For this review, take the finished solid that the model builds, in its own axes (mm). A direction names the side the tool comes from. Round coordinates to 2 decimals unless told otherwise and drop trailing zeros. Order: outer loops, then holes, each group sorted by start corner. A loop starts at its lowest first (then second) coordinate and runs counter-clockwise, first axis right, second up. Notation, with made-up numbers: M 44.25,-13 L 94.25,-13 A14 cw 94.25,12 Z; hole C -23.75,30 d6. An arc over 180 degrees is marked long. Answer as a JSON object with one key per item and string values.
from build123d import *

# Parameters (mm, degrees)
SKETCH1_W           = 7
SKETCH1_H           = 7
BOSS_EXTRUDE1_DEPTH = 4
CUT_EXTRUDE1_DEPTH  = 2
SKETCH4_R           = 1.45
CUT_EXTRUDE2_DEPTH  = 2
FILLET1_R           = 2


with BuildPart() as part:
    # Sketch1 → Boss-Extrude1 (new body)
    with BuildSketch(Plane(origin=(0, 0, 0), x_dir=(1, 0, 0), z_dir=(0, 1, 0))):
        Rectangle(SKETCH1_W, SKETCH1_H)
    extrude(amount=BOSS_EXTRUDE1_DEPTH)

    # Sketch2 → Cut-Extrude1 (cut)
    with BuildSketch(Plane(origin=(0, 4, 0), x_dir=(1, 0, 0), z_dir=(0, 1, 0))):
        Polygon((2.598076211, -1.5), (2.598076211, 1.5), (0, 3), (-2.598076211, 1.5), (-2.598076211, -1.5), (0, -3), align=None)
    extrude(amount=-CUT_EXTRUDE1_DEPTH, mode=Mode.SUBTRACT)

    # Sketch4 → Cut-Extrude2 (cut)
    with BuildSketch(Plane(origin=(0, 2, 0), x_dir=(1, 0, 0), z_dir=(0, 1, 0))):
        with Locations(Location((0, 0, 0), (0, 0, 270))):
            Circle(SKETCH4_R)
    extrude(amount=-CUT_EXTRUDE2_DEPTH, mode=Mode.SUBTRACT)

    # Fillet1
    fillet1_edges = [part.edges().sort_by_distance(p)[0] for p in [
        (3.5, 2, 3.5),
        (-3.5, 2, 3.5),
        (-3.5, 2, -3.5),
        (3.5, 2, -3.5),
    ]]
    fillet(fillet1_edges, radius=FILLET1_R)


solid = part.part
1) Machinability: for faces 1 (the flat face through (2.598, 3, 0)), 2 (the flat face through (-3.5, 2, 0)), which of the approach directions +Z, -Z, +X, -X, +Y, -Y give a long, thin tool a straight path to every point of the face, cutting with its end or side? Answer none if there is none.
Geometry check:
{"face 1": "+Y", "face 2": "+Z, -Z, -X, +Y, -Y"}
2) Add section A-A on z = 0. State the section outline as (x, y) points, and give its area (3 significant figures).
Geometry check:
{"outline": "M -3.5,0 L -1.45,0 L -1.45,2 L -2.6,2 L -2.6,4 L -3.5,4 Z; M 1.45,0 L 3.5,0 L 3.5,4 L 2.6,4 L 2.6,2 L 1.45,2 Z", "area": "11.8 mm²"}
3) For L1, parallel to X at y = 0.75, z = 0; L2, parallel to X at y = 2.25, z = -0.75; L3, parallel to Y at x = 1.25, z = 2, list the stretches that pass through material, from the lowest coordinate up.
Geometry check:
{"L1": "x = -3.5 to -1.45, 1.45 to 3.5", "L2": "x = -3.5 to -2.6, 2.6 to 3.5", "L3": "y = 0 to 2"}
4) Add section B-B on y = 1.4. State the section outline as (x, z) points.
Geometry check:
{"outline": "M -3.5,-1.5 A2 ccw -1.5,-3.5 L 1.5,-3.5 A2 ccw 3.5,-1.5 L 3.5,1.5 A2 ccw 1.5,3.5 L -1.5,3.5 A2 ccw -3.5,1.5 Z; hole C 0,0 d2.9"}
5) Mouldability with a two-part tool opening along X and no side actions: class faces 3 (the flat face through (1.1, 2, 1.3)), 4 (the cylindrical face through (-2.93, 2.03, -2.9)), 5 (the flat face through (0, 2, -3.5)) as +X half, -X half, draft (parallel to the pull), parting line (faces both ways), or undercut.
Geometry check:
{"face 3": "undercut", "face 4": "-X half", "face 5": "draft"}
6) Add section C-C on x = 0.75. State the section outline as (y, z) points.
Geometry check:
{"outline": "M 0,-3.5 L 4,-3.5 L 4,-2.57 L 2,-2.57 L 2,-1.24 L 0,-1.24 Z; M 0,1.24 L 2,1.24 L 2,2.57 L 4,2.57 L 4,3.5 L 0,3.5 Z"}
7) Add section D-D on y = 3.45. State the section outline as (x, z) points, and give its area (3 significant figures).
Geometry check:
{"outline": "M -3.5,-1.5 A2 ccw -1.5,-3.5 L 1.5,-3.5 A2 ccw 3.5,-1.5 L 3.5,1.5 A2 ccw 1.5,3.5 L -1.5,3.5 A2 ccw -3.5,1.5 Z; hole M -2.6,-1.5 L 0,-3 L 2.6,-1.5 L 2.6,1.5 L 0,3 L -2.6,1.5 Z", "area": "22.2 mm²"}
8) Insertion check: P1, Ø1.5, axis at x = 1, z = -0.5, coming from the +Y side; P2, Ø3, axis at x = -1.5, z = 1, coming from the -Y side. Each pin has a flat end and moves straight along its axis. Give the tip position at first contact, or say it passes through.
Geometry check:
{"P1": "stops at y = 2", "P2": "stops at y = 0"}
